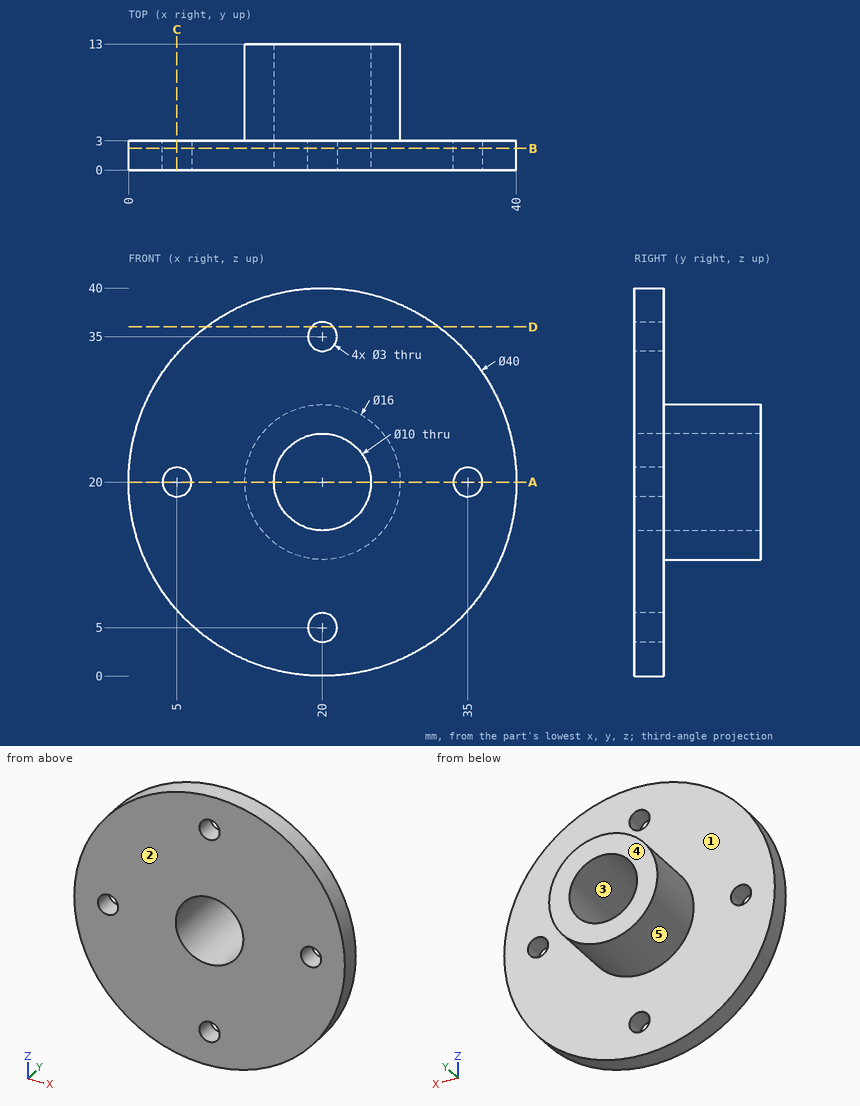
Verification items for this drawing (mm, ordinates from the low corner). A direction names the side the tool comes from. Round coordinates to 2 decimals unless told otherwise and drop trailing zeros. Write each loop counter-clockwise with the first axis right and the second up, starting at its lowest first coordinate (ties: lowest second). Pieces come first, ordered by that corner, then holes. Notation, with made-up numbers: (38, -14.5) - (49, -14.5) arc R27 cw to (49, 10.5) - close; hole circle Ø3 at (-29, -3). An arc over 180 degrees is marked (long way). One line per item, written item: value.
1. Scan lines: L1, parallel to Z at x = 20, y = 2.05; L2, parallel to Z at x = 22, y = 12; L3, parallel to X at y = 2.3, z = 35. Record each from-to range of solid material in increasing order.
The answers:
L1: z = 0 to 3.5, 6.5 to 15, 25 to 33.5, 36.5 to 40
L2: z = 12.25 to 15.42, 24.58 to 27.75
L3: x = 6.77 to 18.5, 21.5 to 33.23
2. Cross-section at C-C on x = 5. Record the boundary of the cut face in (y, z).
The answers:
outline: (0, 6.77) - (3, 6.77) - (3, 18.5) - (0, 18.5) - close; (0, 21.5) - (3, 21.5) - (3, 33.23) - (0, 33.23) - close
3. Set-up check for the marked faces 1 and 2: record each of +Z, -Z, +X, -X, +Y, -Y from which the full face is reachable in a straight line by a thin tool's end or side.
The answers:
face 1: +Y
face 2: +Z, -Z, +X, -X, -Y
4. Depth check by flat-ended pin: pin 1 Ø6 at (x, z) = (8, 7.5) entering from +Y; pin 2 Ø20 at (x, z) = (15, 13.5) entering from +Y; pin 3 Ø1.8 at (x, z) = (20, 35) entering from -Y; pin 4 Ø6 at (x, y) = (24.5, 4) entering from -Z. Enter the tip coordinate at first touch or a pass-through.
The answers:
pin 1: stops at y = 3
pin 2: stops at y = 13
pin 3: passes through
pin 4: stops at z = 0.07
5. Mould release check, pull along Z, two halves, no side actions. Record for the marked faces 3, 4 and 5: released by +Z, released by -Z, zero draft, split by the parting line, or undercut.
The answers:
face 3: undercut
face 4: zero draft
face 5: split by the parting line
6. Cross-section at D-D on z = 36. Record the boundary of the cut face in (x, y), and give its area (3 significant figures).
The answers:
outline: (8, 0) - (18.88, 0) - (18.88, 3) - (8, 3) - close; (21.12, 0) - (32, 0) - (32, 3) - (21.12, 3) - close
area: 65.3 mm^2
7. Cross-section at A-A on z = 20. Record the boundary of the cut face in (x, y).
The answers:
outline: (0, 0) - (3.5, 0) - (3.5, 3) - (0, 3) - close; (6.5, 0) - (15, 0) - (15, 13) - (12, 13) - (12, 3) - (6.5, 3) - close; (25, 0) - (33.5, 0) - (33.5, 3) - (28, 3) - (28, 13) - (25, 13) - close; (36.5, 0) - (40, 0) - (40, 3) - (36.5, 3) - close
8. Cross-section at B-B on y = 2.25. Record the boundary of the cut face in (x, z).
The answers:
outline: circle Ø40 at (20, 20); hole circle Ø3 at (5, 20); hole circle Ø10 at (20, 20); hole circle Ø3 at (20, 5); hole circle Ø3 at (20, 35); hole circle Ø3 at (35, 20)
